```python
from build123d import *

# Parameters (mm, degrees)
SKETCH1_W           = 40
SKETCH1_H           = 35
BOSS_EXTRUDE1_DEPTH = 2
SKETCH2_W           = 2
SKETCH2_H           = 35
BOSS_EXTRUDE2_DEPTH = 38
FILLET1_R           = 3
BOSS_EXTRUDE3_DEPTH = 1.5
BOSS_EXTRUDE4_START = -33.5
BOSS_EXTRUDE4_DEPTH = 1.5


with BuildPart() as part:
    # Sketch1 → Boss-Extrude1 (new body)
    with BuildSketch(Plane.XY):
        Rectangle(SKETCH1_W, SKETCH1_H)
    extrude(amount=BOSS_EXTRUDE1_DEPTH)

    # Sketch2 → Boss-Extrude2 (add)
    with BuildSketch(Plane.XY.offset(2)):
        with Locations((-19, 0)):
            Rectangle(SKETCH2_W, SKETCH2_H)
    extrude(amount=BOSS_EXTRUDE2_DEPTH)

    # Fillet1
    fillet1_edges = [part.edges().sort_by_distance(p)[0] for p in [
        (-18, 0, 2),
        (-19, 17.5, 40),
        (-19, -17.5, 40),
        (-20, 0, 0),
        (20, -17.5, 1),
        (20, 17.5, 1),
    ]]
    fillet(fillet1_edges, radius=FILLET1_R)

    # Sketch3 → Boss-Extrude3 (add)
    with BuildSketch(Plane.XZ.offset(17.5)):
        Polygon((1, 2), (-18, 21), (-18, 16.142135624), (-3.857864376, 2), align=None)
    extrude(amount=-BOSS_EXTRUDE3_DEPTH)

    # Sketch3<2> → Boss-Extrude4 (add)
    with BuildSketch(Plane.XZ.offset(17.5).offset(BOSS_EXTRUDE4_START)):
        Polygon((1, 2), (-18, 21), (-18, 16.142135624), (-3.857864376, 2), align=None)
    extrude(amount=-BOSS_EXTRUDE4_DEPTH)


solid = part.part
```
Read the model definition and answer for the solid it produces. Units are mm, in the model's axes. A direction names the side the tool comes from. Give positions to 0.01 mm unless a question says otherwise; leave off trailing zeros. Loops run counter-clockwise (first coordinate to the right, second up) from the corner with the lowest first, then second, coordinate; pieces in that order, holes last.
Item 1: The part is cut by section B-B (z = 13). Write down the section's boundary in (x, y).
Item 2: The part is cut by section C-C (x = -6). Write down the section's boundary in (y, z), and give its area (3 significant figures).
Item 3: For faces 4 (the flat face through (-10, 16, 11)), 5 (the flat face through (-11.03, -16.76, 9.17)), 6 (the flat face through (-8, -17, 11)), determine the directions among +Z, -Z, +X, -X, +Y, -Y from which every point of the face is accessible in a straight line to the end or side of a thin tool.
Item 4: Find the intervals of material crossed by line 1 along X through (y, z) = (-7, 15); line 2 along Z through (x, y) = (18.5, -7.5); line 3 along Z through (x, y) = (-16.5, 6.5), in increasing order.
Item 5: The part is cut by section D-D (x = 2). Write down the section's boundary in (y, z), and give its area (3 significant figures).
Item 6: This flat-tipped pin is pushed along its axis until it touches: pin 1 Ø17.5 at (x, y) = (-2.5, -6) entering from +Z. Where does it stop, or does it pass through?
Item 7: The mould has two halves that part along Z. Classify faces 1 (the flat face through (-19, 0, 40)), 2 (the flat face through (-11.03, 16.74, 9.17)), 3 (the flat face through (-20, 0, 21)): released by +Z, released by -Z, zero draft, split by the parting line, or undercut.
Item 8: The part is cut by section A-A (y = -12). Write down the section's boundary in (x, z).
Taken from the geometry:
1. outline: (-20, -17.5) - (-18, -17.5) - (-18, 17.5) - (-20, 17.5) - close; (-14.86, -17.5) - (-10, -17.5) - (-10, -16) - (-14.86, -16) - close; (-14.86, 16) - (-10, 16) - (-10, 17.5) - (-14.86, 17.5) - close
2. outline: (-17.5, 0) - (17.5, 0) - (17.5, 2) - (-17.5, 2) - close; (-17.5, 4.14) - (-16, 4.14) - (-16, 9) - (-17.5, 9) - close; (16, 4.14) - (17.5, 4.14) - (17.5, 9) - (16, 9) - close
2. area: 84.6 mm2
3. face 4: +Z, +X
3. face 5: +Y, -Y
3. face 6: +Z, +X, +Y, -Y
4. line 1: x = -20 to -18
4. line 2: z = 0 to 2
4. line 3: z = 0 to 2.4
5. outline: (-17.5, 0) - (17.5, 0) - (17.5, 2) - (-17.5, 2) - close
5. area: 70.0 mm2
6. pin 1: stops at z = 2
7. face 1: released by +Z
7. face 2: undercut
7. face 3: zero draft
8. outline: (-20, 3) arc R3 ccw to (-17, 0) - (20, 0) - (20, 2) - (-15, 2) arc R3 cw to (-18, 5) - (-18, 40) - (-20, 40) - close
